from build123d import *

# Parameters (mm, degrees)
SKETCH1_R                                       = 1.55
SKETCH1_R_2                                     = 1.5
BOSS_EXTRUDE1_DEPTH                             = 11
CUT_EXTRUDE1_DEPTH                              = 6
CSK_FOR_M3_FLAT_HEAD_MACHINE_SCREW1_D           = 2.8
CSK_FOR_M3_FLAT_HEAD_MACHINE_SCREW1_DEPTH       = 10
CSK_FOR_M3_FLAT_HEAD_MACHINE_SCREW1_CSINK_D     = 6.3
CSK_FOR_M3_FLAT_HEAD_MACHINE_SCREW1_CSINK_ANGLE = 90
CSK_FOR_M3_FLAT_HEAD_MACHINE_SCREW1_TIP         = 0.841204867
FILLET1_R                                       = 1


with BuildPart() as part:
    # Sketch1 → Boss-Extrude1 (new body, symmetric)
    with BuildSketch(Plane.XY):
        with BuildLine():
            Line((1.082531755, 9.375), (-3.247595264, 1.875))
            ThreePointArc((-3.247595264, 1.875), (-3.247595264, -1.875), (0, -3.75))
            Line((0, -3.75), (15, -3.75))
            Line((15, -3.75), (15, 1.25))
            Line((15, 1.25), (5.051814855, 1.25))
            Line((5.051814855, 1.25), (7.577722283, 5.625))
            ThreePointArc((7.577722283, 5.625), (6.205127019, 10.747595264), (1.082531755, 9.375))
        make_face()
        Circle(SKETCH1_R, mode=Mode.SUBTRACT)
        with Locations((4.330127019, 7.5)):
            Circle(SKETCH1_R_2, mode=Mode.SUBTRACT)
    extrude(amount=BOSS_EXTRUDE1_DEPTH, both=True)

    # Sketch5 → Cut-Extrude1 (cut, symmetric)
    with BuildSketch(Plane.XY):
        with BuildLine():
            Line((-3.680607966, 2.125), (5.998626937, 18.88992663))
            Line((5.998626937, 18.88992663), (13.359842869, 14.63992663))
            Line((13.359842869, 14.63992663), (3.680607966, -2.125))
            ThreePointArc((3.680607966, -2.125), (-2.125, -3.680607966), (-3.680607966, 2.125))
        make_face()
    extrude(amount=CUT_EXTRUDE1_DEPTH, both=True, mode=Mode.SUBTRACT)

    # CSK for M3 Flat Head Machine Screw1
    with Locations(Plane(origin=(0, 1.25, 0), x_dir=(1, 0, 0), z_dir=(0, 1, 0))):
        with Locations((10.5, 0)):
            CounterSinkHole(CSK_FOR_M3_FLAT_HEAD_MACHINE_SCREW1_D / 2, CSK_FOR_M3_FLAT_HEAD_MACHINE_SCREW1_CSINK_D / 2, depth=CSK_FOR_M3_FLAT_HEAD_MACHINE_SCREW1_DEPTH, counter_sink_angle=CSK_FOR_M3_FLAT_HEAD_MACHINE_SCREW1_CSINK_ANGLE)
            with Locations((0, 0, -(CSK_FOR_M3_FLAT_HEAD_MACHINE_SCREW1_DEPTH + CSK_FOR_M3_FLAT_HEAD_MACHINE_SCREW1_TIP / 2))):  # 118° drill point
                Cone(0, CSK_FOR_M3_FLAT_HEAD_MACHINE_SCREW1_D / 2, CSK_FOR_M3_FLAT_HEAD_MACHINE_SCREW1_TIP, mode=Mode.SUBTRACT)

    # Fillet1
    fillet1_edges = [part.edges().sort_by_distance(p)[0] for p in [
        (2, -3.75, 0),
    ]]
    fillet(fillet1_edges, radius=FILLET1_R)


solid = part.part
Input: part model. Units: mm. Frame: model coordinates. A direction names the side the tool comes from. Coordinates: 2 decimals unless noted, no trailing zeros. Write each loop counter-clockwise with the first axis right and the second up, starting at its lowest first coordinate (ties: lowest second). Pieces come first, ordered by that corner, then holes. Notation, with made-up numbers: M 41.5,29 L 78.5,29 A21 cw 78.5,53 Z; hole C 88,1.25 d4. An arc over 180 degrees is marked long. Answer as a JSON object with one key per item and string values. Group by question number.
(1) Section A-A on y = 7.5. Output: boundary loops of the cut face in (x, z).
(2) Section B-B on z = 0. Output: boundary loops of the cut face in (x, y) (3 decimals).
(3) Section D-D on x = 10.5. Output: boundary loops of the cut face in (y, z), plus the area to 3 significant figures.
(4) Section C-C on y = 0. Output: boundary loops of the cut face in (x, z).
(5) Contact query for flat-ended pins moving along their axis: P1, Ø6, axis at y = 2.5, z = -2.5, coming from the -X side; P2, Ø6, axis at x = 0, z = -8.5, coming from the +Y side; P3, Ø3, axis at x = 8, z = 3.5, coming from the +Y side; P4, Ø2.5, axis at x = 4.33, y = 7.5, coming from the +Z side. Output: stop coordinate, or through.
(6) Ray query, line 1 along X through (y, z) = (7.5, -8.85); line 2 along Z through (x, y) = (3, 10.75); line 3 along X through (y, z) = (0, -8.05). Return the intervals inside material, ascending. Write a range as [from, to].
(7) Mould query, pull axis X, two halves, no side actions, for faces 1 (the face through (4.005, 6.036, 8.465)), 2 (the face through (5, 2, 11)), 3 (the face through (6.276, 10.706, 8.535)). Classes: pulls with the +X half, pulls with the -X half, needs draft (parallel to the pull), parting line crosses it, or undercut.
(8) Set-up query: faces 4 (the face through (4.67, -0.41, 0.08)), 5 (the face through (6.3, 3.41, -8.46)), 6 (the face through (3.59, -3.22, 0.08)). Return all of +Z, -Z, +X, -X, +Y, -Y with unobstructed straight access to the full face (end or side cutting, diameter ignored); none if empty.
Result set:
{
 "1": {"outline": "M 0,-11 L 2.83,-11 L 2.83,-6 L 0,-6 Z; M 0,6 L 2.83,6 L 2.83,11 L 0,11 Z; M 5.83,-11 L 8.08,-11 L 8.08,-6 L 5.83,-6 Z; M 5.83,6 L 8.08,6 L 8.08,11 L 5.83,11 Z"},
 "2": {"outline": "M 3.62,-2.226 A1 ccw 4.472,-3.75 L 9.1,-3.75 L 9.1,-0.5 L 7.35,1.25 L 5.629,1.25 L 3.681,-2.125 A4.25 cw Z; M 11.9,-3.75 L 15,-3.75 L 15,1.25 L 13.65,1.25 L 11.9,-0.5 Z"},
 "3": {"outline": "M -3.75,-11 L 1.25,-11 L 1.25,-3.15 L -0.5,-1.4 L -3.75,-1.4 Z; M -3.75,1.4 L -0.5,1.4 L 1.25,3.15 L 1.25,11 L -3.75,11 Z", "area": "92.9 mm2"},
 "4": {"outline": "M -3.75,-11 L -1.55,-11 L -1.55,-6 L -3.75,-6 Z; M -3.75,6 L -1.55,6 L -1.55,11 L -3.75,11 Z; M 1.55,-11 L 15,-11 L 15,11 L 1.55,11 L 1.55,6 L 4.91,6 L 4.91,-6 L 1.55,-6 Z; hole C 10.5,0 d3.8"},
 "5": {"P1": "stops at x = 4.62", "P2": "stops at y = 11.01", "P3": "stops at y = 1.25", "P4": "passes through"},
 "6": {"line 1": "x = [0, 2.83], [5.83, 8.08]", "line 2": "z = [-11, -6], [6, 11]", "line 3": "x = [-3.75, -1.55], [1.55, 15]"},
 "7": {"face 1": "undercut", "face 2": "needs draft", "face 3": "parting line crosses it"},
 "8": {"face 4": "-X, +Y", "face 5": "+Z, -Z, +X", "face 6": "-X"}
}
